Model file for the job. Use its own axes, mm. Face numbers are marked on the shaded views. A direction names the side the tool comes from. Give positions to 0.01 mm unless a question says otherwise; leave off trailing zeros. Loops run counter-clockwise (first coordinate to the right, second up) from the corner with the lowest first, then second, coordinate; pieces in that order, holes last. Notation, with made-up numbers: (-13, 26) - (-4, 26) arc R33 cw to (-4, 56) - close; hole circle Ø9 at (53, 31.5). An arc over 180 degrees is marked (long way). Use a Markdown table: item, result.
from build123d import *

# Parameters (mm, degrees)
SKETCH1_R           = 25
SKETCH1_R_2         = 12
SKETCH1_R_3         = 6
BOSS_EXTRUDE1_DEPTH = 10


with BuildPart() as part:
    # Sketch1 → Boss-Extrude1 (new body)
    # profile 1 of 3: a face of its own
    with BuildSketch(Plane.XY):
        with Locations((0, 95)):
            Circle(SKETCH1_R)
        Polygon((-10.392304845, 89), (0, 83), (10.392304845, 89), (10.392304845, 101), (0, 107), (-10.392304845, 101), align=None, mode=Mode.SUBTRACT)
    # profile 2 of 3: a face of its own
    with BuildSketch(Plane.XY):
        with BuildLine():
            ThreePointArc((0, 70), (35, 60.621778265), (60.621778265, 35))
            ThreePointArc((60.621778265, 35), (66.215959074, 51.999000215), (82.481329918, 44.535852182))
            ThreePointArc((82.481329918, 44.535852182), (54.13048872, 91.246307211), (7.053536481, 118.98432036))
            ThreePointArc((7.053536481, 118.98432036), (20.016723159, 109.977676522), (25, 95))
            ThreePointArc((25, 95), (17.67766953, 77.32233047), (0, 70))
        make_face()
    # profile 3 of 3: a face of its own
    with BuildSketch(Plane.XY):
        with Locations((71.01408311, 41)):
            Circle(SKETCH1_R_2)
        with Locations((71.01408311, 41)):
            Circle(SKETCH1_R_3, mode=Mode.SUBTRACT)
    extrude(amount=BOSS_EXTRUDE1_DEPTH)


solid = part.part
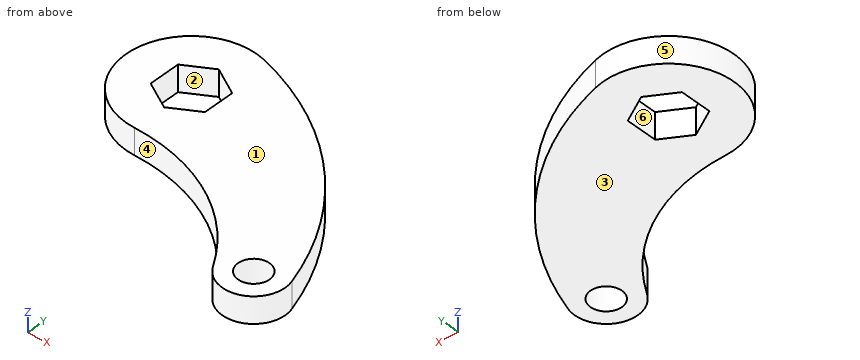
(1) 3-axis set-ups, long thin cutter, end or side, ignore diameter. For the marked faces 1 and 2: which of +Z, -Z, +X, -X, +Y, -Y reach the whole face in a straight line?
Computed:
| item | result |
|---|---|
| face 1 | +Z, +X, -X, +Y, -Y |
| face 2 | +Z, -Z |
(2) Slice it at A-A, the plane x = -4. Write the cut outline in (y, z), plus the area to 3 significant figures.
Computed:
| item | result |
|---|---|
| outline | (70.32, 0) - (85.31, 0) - (85.31, 10) - (70.32, 10) - close; (104.69, 0) - (119.68, 0) - (119.68, 10) - (104.69, 10) - close |
| area | 300 mm² |
(3) Mould opens along Y. For the marked faces 3, 4, 5 and 6 say: pulls with the +Y half, pulls with the -Y half, needs draft (parallel to the pull), parting line crosses it, or undercut.
Computed:
| item | result |
|---|---|
| face 3 | needs draft |
| face 4 | pulls with the -Y half |
| face 5 | parting line crosses it |
| face 6 | undercut |
(4) Slice it at D-D, the plane y = 50.5. Write the cut outline in (x, z).
Computed:
| item | result |
|---|---|
| outline | (48.47, 0) - (80.46, 0) - (80.46, 10) - (48.47, 10) - close |
(5) Pin check, flat tips, straight feed: P1, Ø1, axis at y = 42.5, z = 2, coming from the -X side; P2, Ø7, axis at x = 71.01, y = 41, coming from the +Z side; P3, Ø1, axis at y = 54, z = 7.5, coming from the +X side; P4, Ø8, axis at x = 57.5, y = 39, coming from the +Z side. Stop position of each tip, or through.
Computed:
| item | result |
|---|---|
| P1 | x = 55.24 |
| P2 | through |
| P3 | x = 79.29 |
| P4 | z = 10 |
(6) Drill centre lines: probe 1 along Y at (x, z) = (72.5, 5.5); probe 2 along Y at (x, z) = (8, 8.75); probe 3 along X at (y, z) = (83.5, 6.5). Where is each one in solid material? Low to high. Write a range as [from, to].
Computed:
| item | result |
|---|---|
| probe 1 | [29.09, 35.19], [46.81, 67.45] |
| probe 2 | [69.54, 87.62], [102.38, 118.7] |
| probe 3 | [-22.2, -0.87], [0.87, 61.27] |
(7) Slice it at C-C, the plane y = 95. Write the cut outline in (x, z), plus the area to 3 significant figures.
Computed:
| item | result |
|---|---|
| outline | (-25, 0) - (-10.39, 0) - (-10.39, 10) - (-25, 10) - close; (10.39, 0) - (50.14, 0) - (50.14, 10) - (10.39, 10) - close |
| area | 544 mm² |
(8) Slice it at B-B, the plane z = 5.5. Write the cut outline in (x, y).
Computed:
| item | result |
|---|---|
| outline | (0, 70) arc R70 cw to (60.62, 35) arc R12 ccw to (82.48, 44.54) arc R112 ccw to (7.05, 118.98) arc R25 ccw (long way) to start; hole (-10.39, 89) - (0, 83) - (10.39, 89) - (10.39, 101) - (0, 107) - (-10.39, 101) - close; hole circle Ø12 at (71.01, 41) |
